Work out the finished part from the listing and answer in its coordinate system (mm). A direction names the side the tool comes from. Give positions to 0.01 mm unless a question says otherwise; leave off trailing zeros. Loops run counter-clockwise (first coordinate to the right, second up) from the corner with the lowest first, then second, coordinate; pieces in that order, holes last. Notation, with made-up numbers: M 68.5,8 L 114.5,8 A23 cw 114.5,24 Z; hole C 9,30 d6. An arc over 180 degrees is marked long. Use a Markdown table: item, result.
```python
from build123d import *

# Parameters (mm, degrees)
SKETCH1_W           = 150
SKETCH1_H           = 20
BOSS_EXTRUDE1_DEPTH = 5
SKETCH2_R           = 120.1
CUT_EXTRUDE1_DEPTH  = 3
SKETCH3_R           = 2.3
CUT_EXTRUDE4_DEPTH  = 76.828754441
CHAMFER1_SIZE       = 7


with BuildPart() as part:
    # Sketch1 → Boss-Extrude1 (new body)
    with BuildSketch(Plane(origin=(0, 0, 0), x_dir=(1, 0, 0), z_dir=(0, 1, 0))):
        Rectangle(SKETCH1_W, SKETCH1_H)
    extrude(amount=BOSS_EXTRUDE1_DEPTH)

    # Sketch2 → Cut-Extrude1 (cut)
    with BuildSketch(Plane(origin=(0, 5, 0), x_dir=(1, 0, 0), z_dir=(0, 1, 0))):
        with Locations((0, 114.3)):
            Circle(SKETCH2_R)
    extrude(amount=-CUT_EXTRUDE1_DEPTH, mode=Mode.SUBTRACT)

    # Sketch3 → Cut-Extrude4 (cut, through all)
    with BuildSketch(Plane(origin=(0, 0, 0), x_dir=(1, 0, 0), z_dir=(0, 1, 0))):
        with Locations(Location((-62, 0, 0), (0, 0, 270))):
            Circle(SKETCH3_R)
        with Locations(Location((62, 0, 0), (0, 0, 270))):
            Circle(SKETCH3_R)
    extrude(amount=CUT_EXTRUDE4_DEPTH, mode=Mode.SUBTRACT)

    # Chamfer1
    # the kernel refuses this chamfer: 7 mm, written as the material it takes off along each edge
    with BuildSketch(Plane(origin=(75, 5, 28.001780916), x_dir=(0.02749587661058612, -0.9996219169112968, 0), z_dir=(0, 0, -1)), Plane(origin=(-75, 5, -28.001780916), x_dir=(-0.02749587661058612, -0.9996219169112968, 0), z_dir=(0, 0, 1))) as chamfer1_piece_1:
        Polygon((CHAMFER1_SIZE * 0.999621916911, CHAMFER1_SIZE * 0.0274958766106), (-CHAMFER1_SIZE * 0.0274958766106, CHAMFER1_SIZE * 0.999621916911), (0, 0), align=None)
    extrude(amount=56.003561832, mode=Mode.SUBTRACT)


solid = part.part
```
(1) The mould has two halves that part along X. Classify faces 3 (the flat face through (-1, 0, 0)), 4 (the flat face through (-1, 2, -4)), 5 (the flat face through (71, 2, 0)): released by +X, released by -X, zero draft, split by the parting line, or undercut.
Entries:
| item | result |
|---|---|
| face 3 | zero draft |
| face 4 | undercut |
| face 5 | released by +X |
(2) Which of the six approach directions +Z, -Z, +X, -X, +Y, -Y give full straight-line access (tool end or side, diameter ignored) to faces 1 (the flat face through (-1, 2, 10)), 2 (the cylindrical face through (-0.872, 3.521, 5.797))?
Entries:
| item | result |
|---|---|
| face 1 | +Z, +X, -X, +Y, -Y |
| face 2 | -Z, +Y |
(3) Consider probe 1 along Z at (x, y) = (-62, 1.1); probe 2 along Y at (x, z) = (-43, -7.5); probe 3 along X at (y, z) = (1.95, 0). Determine where each line is inside the solid, lowest interval first. Write a range as [from, to].
Entries:
| item | result |
|---|---|
| probe 1 | z = [-10, -2.3], [2.3, 10] |
| probe 2 | y = [0, 2] |
| probe 3 | x = [-71.05, -64.3], [-59.7, 59.7], [64.3, 71.05] |
(4) A cutting plane is placed at D-D (z = -6). Write down the section's boundary in (x, y).
Entries:
| item | result |
|---|---|
| outline | M -73,0 L 73,0 L 68,5 L 51.91,5 L 51.91,2 L -51.91,2 L -51.91,5 L -68,5 Z |
(5) A cutting plane is placed at C-C (z = 0). Write down the section's boundary in (x, y), and give its area (3 significant figures).
Entries:
| item | result |
|---|---|
| outline | M -73,0 L -64.3,0 L -64.3,5 L -68,5 Z; M -59.7,0 L 59.7,0 L 59.7,5 L 36.87,5 L 36.87,2 L -36.87,2 L -36.87,5 L -59.7,5 Z; M 64.3,0 L 73,0 L 68,5 L 64.3,5 Z |
| area | 438 mm² |
(6) A cutting plane is placed at B-B (x = -62). Write down the section's boundary in (y, z).
Entries:
| item | result |
|---|---|
| outline | M 0,-10 L 5,-10 L 5,-2.3 L 0,-2.3 Z; M 0,2.3 L 5,2.3 L 5,10 L 0,10 Z |
(7) A cutting plane is placed at A-A (y = 3.3). Write down the section's boundary in (x, z).
Entries:
| item | result |
|---|---|
| outline | M -69.7,-10 L -59.54,-10 A120.1 cw 59.54,-10 L 69.7,-10 L 69.7,10 L -69.7,10 Z; hole C -62,0 d4.6; hole C 62,0 d4.6 |
(8) Given P1, Ø1.5, axis at x = -41.5, z = -7.5, coming from the +Y side, flat-ended and moving along its own axis, determine where the tip first touches the part or whether it passes through.
Entries:
| item | result |
|---|---|
| P1 | stops at y = 2 |
